Model file for the job. Use its own axes, mm. A direction names the side the tool comes from. Coordinates: 2 decimals unless noted, no trailing zeros. Write each loop counter-clockwise with the first axis right and the second up, starting at its lowest first coordinate (ties: lowest second). Pieces come first, ordered by that corner, then holes.
Q1. Pin check, flat tips, straight feed: P1, Ø6.5, axis at y = 135, z = -0.5, coming from the -X side; P2, Ø6.5, axis at x = 230, z = 3, coming from the +Y side; P3, Ø6.5, axis at y = 154.5, z = 0.5, coming from the +X side. Stop position of each tip, or through.
Q2. Pull direction Y, two halves, no side cores. Call faces 6 (the cylindrical face through (57.969, -128.456, -0.089)), 7 (the flat face through (-228, -37.338, 0)), 8 (the cylindrical face through (47.91, 137.28, -0.09)), 9 (the flat face through (215.9, -123, 0)): released by +Y, released by -Y, zero draft, split by the parting line, or undercut.
Q3. Band-saw the part on C-C, the plane x = 50.8. Write the cut outline in (y, z) (3 decimals).
Q4. Band-saw the part on D-D, the plane y = -54. Write the cut outline in (x, z).
Q5. Drill centre lines: probe 1 along Y at (x, z) = (50.8, -1) (3 decimals); probe 2 along X at (y, z) = (93.5, -2). Where is each one in solid material? Low to high.
Q6. Band-saw the part on B-B, the plane y = 150.3. Write the cut outline in (x, z) (3 decimals).
Q7. Band-saw the part on A-A, the plane z = 4. Write the cut outline in (x, y) (3 decimals).
Q8. Which spindle directions (+Z, -Z, +X, -X, +Y, -Y) get a long thin tool onto all of the face, cutting with end or side? Do faces 1 (the flat face through (-215.9, -121, 0)), 2 (the flat face through (-228, 37.338, 0)), 3 (the flat face through (228, -37.338, 0)), 4 (the flat face through (-3, 3, -6.35)), 5 (the flat face through (228, 37.338, 0)). Say none if no direction does.
from build123d import *

# Parameters (mm, degrees)
BOSS_EXTRUDE1_DEPTH = 6.35
CAVITY1_START       = -6.35
CAVITY1_OUTLINE_R   = 12.7
CAVITY1_DEPTH       = 12.7
MOVE_FACE_SLOT_BY   = 0.762
MOVE_FACE_SLOT_2_BY = 0.762
MOVE_FACE_SLOT_3_BY = 0.762
MOVE_FACE_SLOT_4_BY = 0.762
MOVE_FACE_SLOT_5_BY = 0.762
MOVE_FACE_SLOT_6_BY = 0.762
FILLET1_R           = 3.175
MOVE_FACE_HOLE_BY   = 0.635
MOVE_FACE_HOLE_2_BY = 0.635


# Read off the part's stored shape, not the designer's step: Cavity1
with BuildPart() as part:
    # Sketch1 → Boss-Extrude1 (new, symmetric)
    with BuildSketch(Plane.XY):
        Polygon((-215.9, -38.1), (-215.9, -203.2), (215.9, -203.2), (215.9, -38.1), (241.3, -38.1), (241.3, 38.1), (215.9, 38.1), (215.9, 203.2), (-215.9, 203.2), (-215.9, 38.1), (-241.3, 38.1), (-241.3, -38.1), align=None)
    extrude(amount=BOSS_EXTRUDE1_DEPTH, both=True)

    # Cavity1 outline → Cavity1 (cut)
    with BuildSketch(Plane.XY.offset(CAVITY1_START)):
        with Locations((50.8, -139.7)):
            Circle(CAVITY1_OUTLINE_R)
        with Locations((50.8, 150.3)):
            Circle(CAVITY1_OUTLINE_R)
    extrude(amount=CAVITY1_DEPTH, mode=Mode.SUBTRACT)

    # Move Face slot: a face moved inward by 0.762
    extrude(part.faces().sort_by_distance((241.3, 0, 0))[0], amount=MOVE_FACE_SLOT_BY, dir=(-1, 0, 0), mode=Mode.SUBTRACT)

    # Move Face slot 2: a face moved inward by 0.762
    extrude(part.faces().sort_by_distance((228.6, 38.1, 0))[0], amount=MOVE_FACE_SLOT_2_BY, dir=(0, -1, 0), mode=Mode.SUBTRACT)

    # Move Face slot 3: a face moved inward by 0.762
    extrude(part.faces().sort_by_distance((-228.6, 38.1, 0))[0], amount=MOVE_FACE_SLOT_3_BY, dir=(0, -1, 0), mode=Mode.SUBTRACT)

    # Move Face slot 4: a face moved inward by 0.762
    extrude(part.faces().sort_by_distance((-241.3, 0, 0))[0], amount=MOVE_FACE_SLOT_4_BY, dir=(1, 0, 0), mode=Mode.SUBTRACT)

    # Move Face slot 5: a face moved inward by 0.762
    extrude(part.faces().sort_by_distance((-228.6, -38.1, 0))[0], amount=MOVE_FACE_SLOT_5_BY, dir=(0, 1, 0), mode=Mode.SUBTRACT)

    # Move Face slot 6: a face moved inward by 0.762
    extrude(part.faces().sort_by_distance((228.6, -38.1, 0))[0], amount=MOVE_FACE_SLOT_6_BY, dir=(0, 1, 0), mode=Mode.SUBTRACT)

    # Fillet1
    fillet1_edges = [part.edges().sort_by_distance(p)[0] for p in [
        (215.9, -37.338, 0),
        (240.538, -37.338, 0),
        (240.538, 37.338, 0),
        (215.9, 37.338, 0),
        (-215.9, 37.338, 0),
        (-240.538, 37.338, 0),
        (-240.538, -37.338, 0),
        (-215.9, -37.338, 0),
    ]]
    fillet(fillet1_edges, radius=FILLET1_R)

    # Move Face hole: a curved face moved inward by 0.635
    add(Solid.thicken(part.faces().sort_by_distance((38.1, -139.7, 0))[0], -MOVE_FACE_HOLE_BY), mode=Mode.SUBTRACT)

    # Move Face hole 2: a curved face moved inward by 0.635
    add(Solid.thicken(part.faces().sort_by_distance((38.1, 150.3, 0))[0], -MOVE_FACE_HOLE_2_BY), mode=Mode.SUBTRACT)


solid = part.part
Answer sheet:
1. P1: stops at x = -215.9
1. P2: stops at y = 37.34
1. P3: stops at x = 215.9
2. face 6: undercut
2. face 7: released by -Y
2. face 8: undercut
2. face 9: zero draft
3. outline: (-203.2, -6.35) - (-153.035, -6.35) - (-153.035, 6.35) - (-203.2, 6.35) - close; (-126.365, -6.35) - (136.965, -6.35) - (136.965, 6.35) - (-126.365, 6.35) - close; (163.635, -6.35) - (203.2, -6.35) - (203.2, 6.35) - (163.635, 6.35) - close
4. outline: (-215.9, -6.35) - (215.9, -6.35) - (215.9, 6.35) - (-215.9, 6.35) - close
5. probe 1: y = -203.2 to -153.035, -126.365 to 136.965, 163.635 to 203.2
5. probe 2: x = -215.9 to 215.9
6. outline: (-215.9, -6.35) - (37.465, -6.35) - (37.465, 6.35) - (-215.9, 6.35) - close; (64.135, -6.35) - (215.9, -6.35) - (215.9, 6.35) - (64.135, 6.35) - close
7. outline: (-240.538, -34.163) arc R3.175 ccw to (-237.363, -37.338) - (-219.075, -37.338) arc R3.175 cw to (-215.9, -40.513) - (-215.9, -203.2) - (215.9, -203.2) - (215.9, -40.513) arc R3.175 cw to (219.075, -37.338) - (237.363, -37.338) arc R3.175 ccw to (240.538, -34.163) - (240.538, 34.163) arc R3.175 ccw to (237.363, 37.338) - (219.075, 37.338) arc R3.175 cw to (215.9, 40.513) - (215.9, 203.2) - (-215.9, 203.2) - (-215.9, 40.513) arc R3.175 cw to (-219.075, 37.338) - (-237.363, 37.338) arc R3.175 ccw to (-240.538, 34.163) - close; hole circle Ø26.67 at (50.8, -139.7); hole circle Ø26.67 at (50.8, 150.3)
8. face 1: +Z, -Z, -X, -Y
8. face 2: +Z, -Z, -X, +Y
8. face 3: +Z, -Z, +X, -Y
8. face 4: -Z, +X, -X, +Y, -Y
8. face 5: +Z, -Z, +X, +Y
